from build123d import *

# Parameters (mm, degrees)
F0_W     = 200
F0_H     = 80
F0_W_2   = 98
F0_H_2   = 18
F0_H_3   = 5
F0_W_3   = 11
F1_DEPTH = 10
F2_DEPTH = 20
F3_DEPTH = 31
F4_DEPTH = 128


# Not quite as in the source:
# - a feature names something its author has since deleted; it is built from what else it names


with BuildPart() as f1:
    # F0 (on Top) → F1 (new body)
    with BuildSketch(Plane.XY):
        Rectangle(F0_W, F0_H)
        Polygon((80, 14), (80, -14), (49, -14), (49, -14.0508310869), (-49, -14.0508310869), (-49, -14), (-80, -14), (-80, 14), (-49, 14), (-49, 14.0508310869), (49, 14.0508310869), (49, 14), align=None, mode=Mode.SUBTRACT)
        Rectangle(F0_W_2, F0_H_2)
        Polygon((49, -14), (80, -14), (80, 14), (49, 14), (49, 9), (60, 9), (60, -9), (49, -9), align=None)
        Polygon((-80, -14), (-49, -14), (-49, -9), (-60, -9), (-60, 9), (-49, 9), (-49, 14), (-80, 14), align=None)
        with Locations((0, -11.5)):
            Rectangle(F0_W_2, F0_H_3)
        with Locations((0, 11.5)):
            Rectangle(F0_W_2, F0_H_3)
        with Locations((54.5, 0)):
            Rectangle(F0_W_3, F0_H_2)
        with Locations((-54.5, 0)):
            Rectangle(F0_W_3, F0_H_2)
    extrude(amount=F1_DEPTH)

    # F0 (on Top) → F2 (join)
    with BuildSketch(Plane.XY):
        Polygon((-80, -14), (-49, -14), (-49, -9), (-60, -9), (-60, 9), (-49, 9), (-49, 14), (-80, 14), align=None)
        with Locations((-54.5, 0)):
            Rectangle(F0_W_3, F0_H_2)
        Rectangle(F0_W_2, F0_H_2)
        with Locations((54.5, 0)):
            Rectangle(F0_W_3, F0_H_2)
        Polygon((49, -14), (80, -14), (80, 14), (49, 14), (49, 9), (60, 9), (60, -9), (49, -9), align=None)
        with Locations((0, -11.5)):
            Rectangle(F0_W_2, F0_H_3)
        with Locations((0, 11.5)):
            Rectangle(F0_W_2, F0_H_3)
    extrude(amount=F2_DEPTH)

    # F0 (on Top) → F3 (join)
    with BuildSketch(Plane.XY):
        Polygon((-80, -14), (-49, -14), (-49, -9), (-60, -9), (-60, 9), (-49, 9), (-49, 14), (-80, 14), align=None)
        with Locations((0, 11.5)):
            Rectangle(F0_W_2, F0_H_3)
        with Locations((0, -11.5)):
            Rectangle(F0_W_2, F0_H_3)
        Polygon((49, -14), (80, -14), (80, 14), (49, 14), (49, 9), (60, 9), (60, -9), (49, -9), align=None)
    extrude(amount=F3_DEPTH)

    # F0 (on Top) → F4 (join)
    with BuildSketch(Plane.XY):
        Polygon((-80, -14), (-49, -14), (-49, -9), (-60, -9), (-60, 9), (-49, 9), (-49, 14), (-80, 14), align=None)
        Polygon((49, -14), (80, -14), (80, 14), (49, 14), (49, 9), (60, 9), (60, -9), (49, -9), align=None)
    extrude(amount=F4_DEPTH)


solid = f1.part
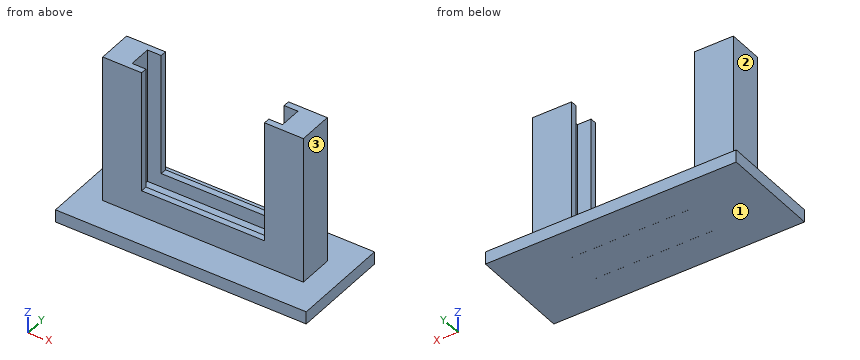
Verification items for the finished model (mm, model axes). Face numbers are marked on the shaded views. A direction names the side the tool comes from. Give positions to 0.01 mm unless a question says otherwise; leave off trailing zeros. Write each loop counter-clockwise with the first axis right and the second up, starting at its lowest first coordinate (ties: lowest second). Pieces come first, ordered by that corner, then holes. Notation, with made-up numbers: M -36,47.25 L -14,47.25 A16 cw -14,52.25 Z; hole C -18,30 d10. An arc over 180 degrees is marked long. Use CSV: the item, a comma, the result in double quotes.
1) Access from +Z, -Z, +X, -X, +Y, -Y to the whole of each face (thin tool, end or side, straight path). Record for the marked faces 1, 2 and 3.
Final values:
face 1,"-Z, +X, -X, +Y, -Y"
face 2,"+Z, -X, +Y, -Y"
face 3,"+Z, +X, +Y, -Y"
2) Cross-section at A-A (z = 103). Enter the section's corners in (x, y), plus the area to 3 significant figures.
Final values:
outline,"M -80,-14 L -49,-14 L -49,-9 L -60,-9 L -60,9 L -49,9 L -49,14 L -80,14 Z; M 49,-14 L 80,-14 L 80,14 L 49,14 L 49,9 L 60,9 L 60,-9 L 49,-9 Z"
area,"1,340 mm²"
3) Cross-section at C-C (z = 22.5). Enter the section's corners in (x, y).
Final values:
outline,"M -80,-14 L 80,-14 L 80,14 L -80,14 Z; hole M -60,-9 L 60,-9 L 60,9 L -60,9 Z"
4) Go/stop test with flat-tipped pins: pin 1 Ø2.5 at (y, z) = (10.5, 75.5) entering from +X; pin 2 Ø2.5 at (y, z) = (-11, 83.5) entering from -X; pin 3 Ø2 at (x, z) = (75.5, 82.5) entering from +Y; pin 4 Ø12 at (x, y) = (-18, -24.5) entering from -Z. Record where each tip stops, or that it passes through.
Final values:
pin 1,"x = 80"
pin 2,"x = -80"
pin 3,"y = 14"
pin 4,"z = 0"
5) Material ranges on line 1 along Y through (x, z) = (53, 114); line 2 along X through (y, z) = (-7, 116); line 3 along Z through (x, y) = (14, -11), recorded low to high.
Final values:
line 1,"-14 to -9, 9 to 14"
line 2,"-80 to -60, 60 to 80"
line 3,"0 to 31"
6) Cross-section at B-B (x = -24.5). Enter the section's corners in (y, z), plus the area to 3 significant figures.
Final values:
outline,"M -40,0 L -14.05,0 L -14.05,10 L -40,10 Z; M -14,0 L 14,0 L 14,31 L 9,31 L 9,20 L -9,20 L -9,31 L -14,31 Z; M 14.05,0 L 40,0 L 40,10 L 14.05,10 Z"
area,"1,190 mm²"
7) Cross-section at D-D (y = 3.5). Enter the section's corners in (x, z).
Final values:
outline,"M -100,0 L 100,0 L 100,10 L 80,10 L 80,128 L 60,128 L 60,20 L -60,20 L -60,128 L -80,128 L -80,10 L -100,10 Z"
